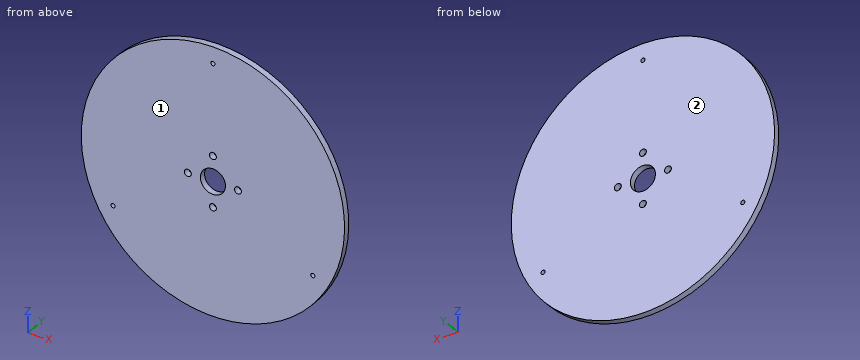
from build123d import *

# Parameters (mm, degrees)
ESQUISSE1_R                               = 105
ESQUISSE1_R_2                             = 10
BOSS_EXTRU_1_DEPTH                        = 5
TROU_POUR_TARAUDAGE_POUR_TROU_TARAUD_M4_D = 3.3
R_P_TITION_CIRCULAIRE1_COUNT              = 3
D_GAGEMENT_M51_D                          = 5.5
R_P_TITION_CIRCULAIRE2_COUNT              = 4


with BuildPart() as part:
    # Esquisse1 → Boss.-Extru.1 (new body)
    with BuildSketch(Plane(origin=(0, 0, 0), x_dir=(1, 0, 0), z_dir=(0, 1, 0))):
        with Locations(Location((0, 0, 0), (0, 0, 270))):
            Circle(ESQUISSE1_R)
        with Locations(Location((0, 0, 0), (0, 0, 270))):
            Circle(ESQUISSE1_R_2, mode=Mode.SUBTRACT)
    extrude(amount=BOSS_EXTRU_1_DEPTH)

    # Trou pour taraudage pour trou taraud_ M4 (through all)
    with Locations(Plane(origin=(0, 5, 0), x_dir=(1, 0, 0), z_dir=(0, 1, 0))):
        with Locations((0, -92)):
            trou_pour_taraudage_pour_trou_taraud_m4 = Hole(TROU_POUR_TARAUDAGE_POUR_TROU_TARAUD_M4_D / 2)

    # R_p_tition circulaire1: Trou pour taraudage pour trou taraud_ M4 ×3 about axis
    r_p_tition_circulaire1_axis = Axis((0, 0, 0), (0, 1, 0))
    for i in range(1, R_P_TITION_CIRCULAIRE1_COUNT):
        add(trou_pour_taraudage_pour_trou_taraud_m4.rotate(r_p_tition_circulaire1_axis, i * 360 / R_P_TITION_CIRCULAIRE1_COUNT), mode=Mode.SUBTRACT)

    # D_gagement M51 (through all)
    with Locations(Plane(origin=(0, 5, 0), x_dir=(1, 0, 0), z_dir=(0, 1, 0))):
        with Locations((0, -20)):
            d_gagement_m51 = Hole(D_GAGEMENT_M51_D / 2)

    # R_p_tition circulaire2: D_gagement M51 ×4 about axis
    r_p_tition_circulaire2_axis = Axis((0, 0, 0), (0, 1, 0))
    for i in range(1, R_P_TITION_CIRCULAIRE2_COUNT):
        add(d_gagement_m51.rotate(r_p_tition_circulaire2_axis, i * 360 / R_P_TITION_CIRCULAIRE2_COUNT), mode=Mode.SUBTRACT)


solid = part.part
Could you check a few things on this model? Use its own coordinates, in mm. Face numbers are marked on the shaded views. Round coordinates to 2 decimals unless told otherwise and drop trailing zeros. Loops run counter-clockwise (first coordinate to the right, second up) from the corner with the lowest first, then second, coordinate; pieces in that order, holes last. Notation, with made-up numbers: (80, 38) -> (125, 38) arc R20 ccw to (125, 64) -> close; hole circle Ø7 at (54.25, 88). An arc over 180 degrees is marked (long way). Use CSV: the item, a comma, the result in double quotes.
(1) Suppose I cut it at B-B on y = 1.2. Give the number of separate pieces and of enclosed holes in the cut face, plus the area to 3 significant figures.
Return value:
separate pieces,"1"
enclosed holes,"8"
area,"34,200 mm²"
(2) Will these pins go through, and if not, where does the flat tip stop? pin 1 Ø2 at (x, y) = (-69.5, 2.5) entering from +Z; pin 2 Ø3 at (y, z) = (4, -16.5) entering from +X; pin 3 Ø2 at (x, z) = (0, 92) entering from +Y; pin 4 Ø3 at (y, z) = (3.5, -83.5) entering from +X.
Return value:
pin 1,"stops at z = 79.58"
pin 2,"stops at x = 103.92"
pin 3,"passes through"
pin 4,"stops at x = 65.58"
(3) Suppose I cut it at A-A on z = 0. Write out the boundary of the cut face in (x, y), plus the area to 3 significant figures.
Return value:
outline,"(-105, 0) -> (-22.75, 0) -> (-22.75, 5) -> (-105, 5) -> close; (-17.25, 0) -> (-10, 0) -> (-10, 5) -> (-17.25, 5) -> close; (10, 0) -> (17.25, 0) -> (17.25, 5) -> (10, 5) -> close; (22.75, 0) -> (105, 0) -> (105, 5) -> (22.75, 5) -> close"
area,"895 mm²"
(4) If we mould it in two halves opening along Y, with no side actions, what happens to the marked faces 1 and 2? For each: +Y half, -Y half, draft (parallel to the pull), parting line (faces both ways), or undercut.
Return value:
face 1,"-Y half"
face 2,"+Y half"
(5) If I drill on probe 1 along X at (y, z) = (3.4, 0); probe 2 along X at (y, z) = (3.5, 8.5); probe 3 along X at (y, z) = (2.5, 20), over which ranges is the centre line in solid material (lowest first)? Write a range as [from, to].
Return value:
probe 1,"x = [-105, -22.75], [-17.25, -10], [10, 17.25], [22.75, 105]"
probe 2,"x = [-104.66, -5.27], [5.27, 104.66]"
probe 3,"x = [-103.08, -2.75], [2.75, 103.08]"
(6) Suppose I cut it at C-C on x = 20. Write out the boundary of the cut face in (y, z).
Return value:
outline,"(0, -103.08) -> (5, -103.08) -> (5, -2.75) -> (0, -2.75) -> close; (0, 2.75) -> (5, 2.75) -> (5, 103.08) -> (0, 103.08) -> close"
(7) Suppose I cut it at D-D on x = -36. Write out the boundary of the cut face in (y, z), plus the area to 3 significant figures.
Return value:
outline,"(0, -98.64) -> (5, -98.64) -> (5, 98.64) -> (0, 98.64) -> close"
area,"986 mm²"
